Part model, mm, in its own coordinate system. Round coordinates to 2 decimals unless told otherwise and drop trailing zeros. Write each loop counter-clockwise with the first axis right and the second up, starting at its lowest first coordinate (ties: lowest second). Pieces come first, ordered by that corner, then holes. Notation, with made-up numbers: (2.25, 40) -> (19.25, 40) arc R21 cw to (19.25, 65) -> close; hole circle Ø7 at (83, -22.5). An arc over 180 degrees is marked (long way). Use CSV: the item, a comma, the result in double quotes. Start each with the question number.
(1) Probe line 1 (X direction, y = 60, z = 1); line 2 (Y direction, x = 0, z = 2.15); line 3 (Y direction, x = -70, z = 2.1). List the from-to ranges inside material, lowest first. Write a range as [from, to].
(2) Saw through at C-C (z = 0.9). Count the separate pieces of the cut face and the enclosed holes in it, plus the area to 3 significant figures.
(3) Drop a flat-ended pin along its axis: pin 1 (3.5 mm diameter, centred on x = -20, y = 31, fed in from +Z) (3 decimals). Give the stop position or say it passes through.
(4) Saw through at B-B (x = 7.5). Give the cut face in (y, z) (3 decimals), plus the area to 3 significant figures.
(5) Saw through at A-A (y = 13.5). Give the cut face in (x, z) (3 decimals).
Autodesk Inventor part; units mm, degrees
ref_plane "YZ Plane" through (0, 0, 0) normal (1, 0, 0) x (0, 1, 0)
ref_plane "XZ Plane" through (0, 0, 0) normal (0, 1, 0) x (-1, 0, 0)
ref_plane "XY Plane" through (0, 0, 0) normal (0, 0, 1) x (1, 0, 0)
sketch "Sketch1" plane through (0, 0, 0) normal (0, 0, 1) x (1, 0, 0)
  line L0 (-75, 65) -> (75, 65)
  line L1 (75, 65) -> (75, -35)
  line L2 (75, -35) -> (-75, -35)
  line L3 (-75, -35) -> (-75, 65)
  point P0 (0, 0)
  dimension "d0" = 150
  dimension "d1" = 100
  dimension "d26" = 75
  dimension "d27" = 65
extrude "Extrusion1" add sketch "Sketch1" along normal blind 3.175
sketch "Sketch2" plane through (0, 0, 3.175) normal (0, 0, 1) x (1, 0, 0)
  line L0 (75, 65) -> (-75, 65)
  line L1 (-75, 65) -> (-75, -35)
  line L2 (75, -35) -> (75, 65)
  line L3 (-75, -35) -> (75, -35)
  point P0 (0, 0)
  point P1 (-70, 60)
  point P2 (70, 60)
  point P3 (70, -30)
  point P4 (-70, -30)
  dimension "d4" = 5
  dimension "d5" = 5
  dimension "d6" = 5
  dimension "d7" = 5
  dimension "d8" = 5
  dimension "d9" = 5
  dimension "d10" = 5
  dimension "d11" = 5
hole "Hole1" at (-70, 60, 3.175) at (70, 60, 3.175) at (70, -30, 3.175) at (-70, -30, 3.175) direction (0, 0, -1) diameter 3 end through all countersink diameter 4 countersink angle 90
fillet "Fillet1" radius 5 4 edges at (-75, 65, 1.5875) (75, 65, 1.5875) (75, -35, 1.5875) (-75, -35, 1.5875)
sketch "Sketch4" plane through (0, 0, 0) normal (0, 0, -1) x (-1, 0, 0)
  circle A0 centre (0, 0) radius 3.5
  circle A1 centre (0, 8.5) radius 1.5
  circle A2 centre (0, -8.5) radius 1.5
  dimension "d35" = 7
  dimension "d36" = 8.5
  dimension "d37" = 8.5
  dimension "d38" = 3
  dimension "d39" = 3
  dimension "d40" = 0
  dimension "d41" = 0
extrude "Extrusion3" cut sketch "Sketch4" against normal up to next
sketch "Sketch5" plane through (0, 0, 0) normal (0, 0, -1) x (-1, 0, 0)
  line L0 (5.9999, -30) -> (5.9999, 8.0565) construction
  line L1 (11.1182, -28.5024) -> (4.5396, 8.8062) construction
  line L2 (15.8986, -26.1386) -> (3.2654, 8.571) construction
  line L3 (20.1961, -22.9808) -> (2.6287, 7.447) construction
  line L4 (23.8798, -19.1247) -> (2.1665, 6.7525) construction
  line L5 (-70, -35) -> (70, -35)
  line L6 (75, -30) -> (75, 60)
  line L7 (10.5712, -25.4002) -> (13.7361, -24.8422)
  line L8 (14.8213, -23.1786) -> (18.4034, -21.8748) construction
  line L9 (18.6211, -20.2528) -> (20.9099, -18.9314) construction
  line L10 (21.855, -16.7116) -> (23.791, -15.0872) construction
  arc A0 (11.1499, -20.35) -> (17.4375, -15.3092) centre (0.0019, -0.0027) ccw construction
  arc A1 (17.4375, -15.3092) -> (21.6221, -8.422) centre (0.0014, -0.0005) ccw construction
  arc A2 (11.1499, -26.85) -> (19.6607, -21.4172) centre (0.0018, -0.0031) ccw construction
  arc A3 (19.6607, -21.4172) -> (25.8002, -13.4013) centre (0.0012, -0.0006) ccw construction
  arc A4 (11.1499, -20.35) -> (21.6221, -8.422) centre (-0.0011, 0.001) ccw construction
  arc A5 (11.6424, -21.2489) -> (22.5772, -8.794) centre (-0.0011, 0.001) ccw
  arc A6 (10.6574, -19.4511) -> (20.667, -8.05) centre (-0.0011, 0.001) ccw
  arc A7 (10.6574, -19.4511) -> (11.6424, -21.2489) centre (11.1499, -20.35) ccw
  arc A8 (22.5772, -8.794) -> (20.667, -8.05) centre (21.6221, -8.422) ccw
  arc A9 (11.1499, -26.85) -> (25.8002, -13.4013) centre (-0.0009, 0.001) ccw construction
  arc A10 (11.543, -27.7966) -> (26.7098, -13.8738) centre (-0.0009, 0.001) ccw
  arc A11 (10.7568, -25.9034) -> (24.8906, -12.9288) centre (-0.0009, 0.001) ccw
  arc A12 (10.7568, -25.9034) -> (11.543, -27.7966) centre (11.1499, -26.85) ccw
  arc A13 (26.7098, -13.8738) -> (24.8906, -12.9288) centre (25.8002, -13.4013) ccw
  line L11 (0, -12.0487) -> (0, -35) construction
  arc A14 (-22.5772, -8.794) -> (-11.6424, -21.2489) centre (0.0011, 0.001) ccw
  arc A15 (-20.667, -8.05) -> (-10.6574, -19.4511) centre (0.0011, 0.001) ccw
  arc A16 (-11.6424, -21.2489) -> (-10.6574, -19.4511) centre (-11.1499, -20.35) ccw
  arc A17 (-20.667, -8.05) -> (-22.5772, -8.794) centre (-21.6221, -8.422) ccw
  arc A18 (-26.7098, -13.8738) -> (-11.543, -27.7966) centre (0.0009, 0.001) ccw
  arc A19 (-24.8906, -12.9288) -> (-10.7568, -25.9034) centre (0.0009, 0.001) ccw
  arc A20 (-11.543, -27.7966) -> (-10.7568, -25.9034) centre (-11.1499, -26.85) ccw
  arc A21 (-24.8906, -12.9288) -> (-26.7098, -13.8738) centre (-25.8002, -13.4013) ccw
  point P0 (0, 0)
  point P1 (15.643, -24.5059)
  point P2 (14.5143, -18.1047)
  point P3 (23.0811, -17.6778)
  point P4 (19.8311, -12.0486)
  dimension "d48" = 5.15
  dimension "d50" = 3.15
  dimension "d51" = 6.5
  dimension "d52" = 5.15
  dimension "d53" = 5.15
  dimension "d54" = 3.15
  dimension "d55" = 0
  dimension "d56" = 5.15
  dimension "d57" = 6.5
  dimension "d58" = 5.15
  dimension "d59" = 5.15
  dimension "d60" = 3.15
  dimension "d61" = 0
  dimension "d62" = 6.5
  dimension "d63" = 5.15
  dimension "d64" = 5.15
  dimension "d65" = 3.15
  dimension "d66" = 0
  dimension "d67" = 6.5
  dimension "d68" = 5.15
  dimension "d69" = 5.15
  dimension "d70" = 3.15
  dimension "d71" = 0
  dimension "d72" = 6.5
  dimension "d73" = 2.05
  dimension "d74" = 2.05
  dimension "d75" = 22.9513
extrude "Extrusion4" cut sketch "Sketch5" against normal through all
sketch "Sketch8" plane through (0, 0, 3.175) normal (0, 0, 1) x (1, 0, 0)
  point P0 (0, 0)
  point P1 (-7.5, 13.5)
  point P2 (7.5, 13.5)
  point P3 (0, -15)
  dimension "d78" = 7.5
  dimension "d79" = 15
  dimension "d80" = 13.5
  dimension "d81" = 13.5
  dimension "d82" = 15
  dimension "d83" = 0
hole "Hole2" at (-7.5, 13.5, 3.175) at (7.5, 13.5, 3.175) at (0, -15, 3.175) direction (0, 0, -1) diameter 3 end through all countersink diameter 4 countersink angle 90
sketch "Sketch9" plane through (0, 0, 3.175) normal (0, 0, 1) x (1, 0, 0)
  line L0 (70, 65) -> (-70, 65)
  line L1 (-75, 60) -> (-75, -30)
  point P0 (0, 0)
  point P1 (-20, 31)
  point P2 (-20, 24)
  point P3 (20, 24)
  point P4 (20, 31)
  dimension "d91" = 40
  dimension "d92" = 34
  dimension "d93" = 7
  dimension "d94" = 7
  dimension "d95" = 34
  dimension "d96" = 55
  dimension "d97" = 55
  dimension "d98" = 40
hole "Hole3" at (-20, 31, 3.175) at (-20, 24, 3.175) at (20, 24, 3.175) at (20, 31, 3.175) direction (0, 0, -1) diameter 3 end through all countersink diameter 4 countersink angle 90
properties part number "SheetPot"
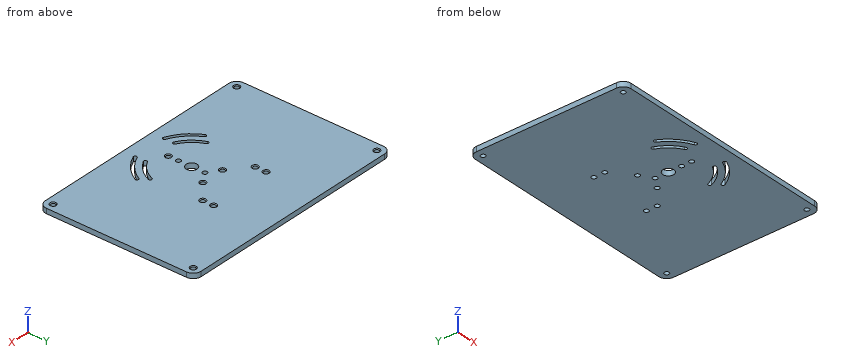
Answers:
1,line 1,"x = [-75, -71.5], [-68.5, 68.5], [71.5, 75]"
1,line 2,"y = [-35, -16.5], [-13.5, -10], [-7, -3.5], [3.5, 7], [10, 65]"
1,line 3,"y = [-35, -31.5], [-28.5, 58.5], [61.5, 65]"
2,separate pieces,"1"
2,enclosed holes,"18"
2,area,"14,700 mm²"
3,pin 1,"stops at z = 2.925"
4,outline,"(-35, 0) -> (12, 0) -> (12, 2.675) -> (11.5, 3.175) -> (-35, 3.175) -> close; (15, 0) -> (65, 0) -> (65, 3.175) -> (15.5, 3.175) -> (15, 2.675) -> close"
4,area,"308 mm²"
5,outline,"(-75, 0) -> (-9, 0) -> (-9, 2.675) -> (-9.5, 3.175) -> (-75, 3.175) -> close; (-6, 0) -> (6, 0) -> (6, 2.675) -> (5.5, 3.175) -> (-5.5, 3.175) -> (-6, 2.675) -> close; (9, 0) -> (75, 0) -> (75, 3.175) -> (9.5, 3.175) -> (9, 2.675) -> close"
